The model under review builds one solid part; all positions refer to its coordinate system, in mm. A direction names the side the tool comes from. Round coordinates to 2 decimals unless told otherwise and drop trailing zeros. Loops run counter-clockwise (first coordinate to the right, second up) from the corner with the lowest first, then second, coordinate; pieces in that order, holes last. Notation, with made-up numbers: (-19, 37) -> (37, 37) arc R12 ccw to (37, 58) -> close; hole circle Ø11 at (-32, 55). An arc over 180 degrees is marked (long way). Use a Markdown table: item, result. Add a question column.
1) Mouldability with a two-part tool opening along Y and no side actions: class faces 1 (the flat face through (39, -2.5, 25)), 2 (the flat face through (0, 41, 20)), 3 (the cylindrical face through (39.584, -12.465, 10.14)), 4 (the cylindrical face through (0.88, -41.49, 35.07)) as released by +Y, released by -Y, zero draft, split by the parting line, or undercut.
2) For faces 5 (the cylindrical face through (-0.86, 40.49, 25.07)), 6 (the flat face through (-3, -41, 20)), 7 (the flat face through (-39, 0, 10)), list the 3-axis set-ups (+Z, -Z, +X, -X, +Y, -Y) from which the entire face can be reached by the end or side of a thin tool; tool diameter is ignored.
3) Consider section A-A on x = 0. Give the boundary of the cut face in (y, z), plus the area to 3 significant figures.
4) Consider section B-B on y = 0. Give the boundary of the cut face in (x, z).
5) Insertion check: pin 1 (5 mm diameter, centred on y = -19, z = 16.5, fed in from +X); pin 2 (1 mm diameter, centred on x = -31, z = 25, fed in from +Y); pin 3 (2 mm diameter, centred on y = 28, z = 33.5, fed in from +X). Each pin has a flat end and moves straight along its axis. Give the tip position at first contact, or say it passes through.
6) Wall thickness on probe 1 along Y at (x, z) = (0, 27); probe 2 along Y at (x, z) = (0, 13); probe 3 along X at (y, z) = (25, 29): over which ranges is each line inside the solid? List them lowest first.
7) Consider section C-C on x = -30. Give the boundary of the cut face in (y, z), plus the area to 3 significant figures.
from build123d import *

# Parameters (mm, degrees)
F2_W     = 100
F2_H     = 5
F3_DEPTH = 30


with BuildPart() as f1:
    # F0 (on Front) → F1 (revolve)
    with BuildSketch(Plane.XZ):
        Polygon((0, 5), (0, 0), (41.5, 0), (41.5, 20), (40.5, 20), (40.5, 30), (41.5, 30), (41.5, 40), (36.5, 40), (36.5, 5), align=None)
    revolve(axis=Axis((0, 0, 2.5), (0, 0, -1)))

    # F2 (on face) → F3 (cut)
    with BuildSketch(Plane.XY.offset(40)):
        Rectangle(F2_W, F2_H)
    extrude(amount=-F3_DEPTH, mode=Mode.SUBTRACT)


solid = f1.part
Result set:
| question | item | result |
|---|---|---|
| 1 | face 1 | undercut |
| 1 | face 2 | zero draft |
| 1 | face 3 | split by the parting line |
| 1 | face 4 | released by -Y |
| 2 | face 5 | +Y |
| 2 | face 6 | -Y |
| 2 | face 7 | +Z, +X, -X |
| 3 | outline | (-41.5, 0) -> (41.5, 0) -> (41.5, 20) -> (40.5, 20) -> (40.5, 30) -> (41.5, 30) -> (41.5, 40) -> (36.5, 40) -> (36.5, 5) -> (-36.5, 5) -> (-36.5, 40) -> (-41.5, 40) -> (-41.5, 30) -> (-40.5, 30) -> (-40.5, 20) -> (-41.5, 20) -> close |
| 3 | area | 745 mm2 |
| 4 | outline | (-41.5, 0) -> (41.5, 0) -> (41.5, 10) -> (36.5, 10) -> (36.5, 5) -> (-36.5, 5) -> (-36.5, 10) -> (-41.5, 10) -> close |
| 5 | pin 1 | x = 38.08 |
| 5 | pin 2 | y = 26.65 |
| 5 | pin 3 | x = 31.52 |
| 6 | probe 1 | -40.5 to -36.5, 36.5 to 40.5 |
| 6 | probe 2 | -41.5 to -36.5, 36.5 to 41.5 |
| 6 | probe 3 | -31.86 to -26.59, 26.59 to 31.86 |
| 7 | outline | (-28.67, 0) -> (28.67, 0) -> (28.67, 20) -> (27.21, 20) -> (27.21, 30) -> (28.67, 30) -> (28.67, 40) -> (20.79, 40) -> (20.79, 5) -> (-20.79, 5) -> (-20.79, 40) -> (-28.67, 40) -> (-28.67, 30) -> (-27.21, 30) -> (-27.21, 20) -> (-28.67, 20) -> close |
| 7 | area | 809 mm2 |
